For this review, take the finished solid that the model builds, in its own axes (mm). A direction names the side the tool comes from. Round coordinates to 2 decimals unless told otherwise and drop trailing zeros. Order: outer loops, then holes, each group sorted by start corner. A loop starts at its lowest first (then second) coordinate and runs counter-clockwise, first axis right, second up.
from build123d import *

# Parameters (mm, degrees)
SKETCH1_R           = 4
BOSS_EXTRUDE1_DEPTH = 12.5
SKETCH2_R           = 10
CUT_EXTRUDE1_DEPTH  = 15
SKETCH3_W           = 24
SKETCH3_H           = 31
CUT_EXTRUDE2_DEPTH  = 10


with BuildPart() as part:
    # Sketch1 → Boss-Extrude1 (new, symmetric)
    with BuildSketch(Plane(origin=(0, 0, 0), x_dir=(1, 0, 0), z_dir=(0, 1, 0))):
        Polygon((-40.5, -10), (-40, -10), (-40, -25), (40, -25), (40, -10), (40.5, -10), (40.5, 10), (-40.5, 10), align=None)
        with Locations(Location((-25, 0, 0), (0, 0, 270))):
            Circle(SKETCH1_R, mode=Mode.SUBTRACT)
        with Locations(Location((25, 0, 0), (0, 0, 90))):
            Circle(SKETCH1_R, mode=Mode.SUBTRACT)
    extrude(amount=BOSS_EXTRUDE1_DEPTH, both=True)

    # Sketch2 → Cut-Extrude1 (cut)
    with BuildSketch(Plane.XY.offset(25)):
        with Locations((-27.5, 0)):
            Circle(SKETCH2_R)
        with Locations(Location((27.5, 0, 0), (0, 0, 180))):
            Circle(SKETCH2_R)
    extrude(amount=-CUT_EXTRUDE1_DEPTH, mode=Mode.SUBTRACT)

    # Sketch3 → Cut-Extrude2 (cut)
    with BuildSketch(Plane.XY.offset(25)):
        Rectangle(SKETCH3_W, SKETCH3_H)
    extrude(amount=-CUT_EXTRUDE2_DEPTH, mode=Mode.SUBTRACT)


solid = part.part
(1) Add section C-C on x = 35.5. Give the boundary of the cut face in (y, z), plus the area to 3 significant figures.
(2) Add section B-B on y = 0. Give the boundary of the cut face in (x, z), plus the area to 3 significant figures.
(3) Tool access review of faces 4 (the face through (40, 0, 18)), 5 (the face through (28, 0, 10)), 6 (the face through (0, 0, 15)), 7 (the face through (16, 0, 25)): name each direction out of +Z, -Z, +X, -X, +Y, -Y from which nothing blocks a thin tool from reaching the whole face with its end or side.
(4) Add section D-D on z = 0. Give the boundary of the cut face in (x, y), plus the area to 4 significant figures.
(5) Draft analysis for pull direction Y (two halves, no side actions). For faces 1 (the face through (-1, -12.5, 7)), 2 (the face through (-40, 0, 17)), 3 (the face through (-28, 0, 10)), state which applies: pulls with the +Y half, pulls with the -Y half, needs draft (parallel to the pull), parting line crosses it, or undercut.
(6) Clearance check with flat-ended pins moving along their axes: P1, Ø5, axis at y = 1.5, z = 21.5, coming from the -X side; P2, Ø1, axis at x = -24, y = -8, coming from the +Z side; P3, Ø5, axis at x = -0.5, y = -7.5, coming from the +Z side. State where each tip first meets the part, or that it passes through.
(7) Add section A-A on z = 23.5. Give the boundary of the cut face in (x, y).
(8) Wall thickness on L1, parallel to X at y = -0.25, z = 15.5; L2, parallel to X at y = -5.75, z = 0; L3, parallel to Z at x = 25, y = 0.5: over which ranges is each line inside the solid? List them lowest first.
Here are the results:
1. outline: (-12.5, -10) - (12.5, -10) - (12.5, 25) - (6, 25) - (6, 10) - (-6, 10) - (-6, 25) - (-12.5, 25) - close
1. area: 695 mm2
2. outline: (-40.5, -10) - (40.5, -10) - (40.5, 10) - (40, 10) - (40, 25) - (37.5, 25) - (37.5, 10) - (17.5, 10) - (17.5, 25) - (12, 25) - (12, 15) - (-12, 15) - (-12, 25) - (-17.5, 25) - (-17.5, 10) - (-37.5, 10) - (-37.5, 25) - (-40, 25) - (-40, 10) - (-40.5, 10) - close; hole circle Ø8 at (-25, 0); hole circle Ø8 at (25, 0)
2. area: 1,880 mm2
3. face 4: +Z, +X, +Y, -Y
3. face 5: +Z
3. face 6: +Z, +Y, -Y
3. face 7: +Z, +X, -X, +Y, -Y
4. outline: (-40.5, -12.5) - (-29, -12.5) - (-29, 12.5) - (-40.5, 12.5) - close; (-21, -12.5) - (21, -12.5) - (21, 12.5) - (-21, 12.5) - close; (29, -12.5) - (40.5, -12.5) - (40.5, 12.5) - (29, 12.5) - close
4. area: 1,625 mm2
5. face 1: pulls with the -Y half
5. face 2: needs draft
5. face 3: undercut
6. P1: stops at x = -40
6. P2: stops at z = 10
6. P3: stops at z = 15
7. outline: (-40, -12.5) - (-12, -12.5) - (-12, 12.5) - (-40, 12.5) - close; (12, -12.5) - (40, -12.5) - (40, 12.5) - (12, 12.5) - close; hole circle Ø20 at (-27.5, 0); hole circle Ø20 at (27.5, 0)
8. L1: x = -40 to -37.5, -17.5 to -12, 12 to 17.5, 37.5 to 40
8. L2: x = -40.5 to -29, -21 to 21, 29 to 40.5
8. L3: z = -10 to -4, 4 to 10
